from build123d import *

# Parameters (mm, degrees)
F0_W            = 25.4
F0_H            = 25.4
F1_DEPTH        = 12.7
F2_W            = 23
F2_H            = 23
F2_W_2          = 17
F2_H_2          = 17
F3_DEPTH        = 29.6
F3_COPIES_COUNT = 3
F3_COPIES_ANGLE = 180
F4_R            = 1.5


# Not quite as in the source:
# - a pattern or mirror of a feature is missing from the dataset's text; its kind, count and spacing are read off the source's solid


with BuildPart() as f1:
    # F0 (on Front) → F1 (new body, symmetric)
    with BuildSketch(Plane.XZ):
        Rectangle(F0_W, F0_H)
    extrude(amount=F1_DEPTH, both=True)

    # F2 (on face) → F3 (join)
    with BuildSketch(Plane.XZ.offset(12.7)):
        Rectangle(F2_W, F2_H)
        Rectangle(F2_W_2, F2_H_2, mode=Mode.SUBTRACT)
    f3 = extrude(amount=F3_DEPTH)

    # F3_copies: F3 ×3 about axis
    f3_copies_axis = Axis((0, 0, 0), (0, 0, 1))
    for i in range(1, F3_COPIES_COUNT):
        add(f3.rotate(f3_copies_axis, i * F3_COPIES_ANGLE / (F3_COPIES_COUNT - 1)))

    # F3_copies1: F3 across plane
    add(f3.mirror(Plane(origin=(0, 0, 0), x_dir=(0, -0.7071067812, -0.7071067812), z_dir=(0, 0.7071067812, -0.7071067812))))

    # F4
    f4_edges = [f1.edges().sort_by_distance(p)[0] for p in [
        (11.5, -27.5, 11.5),
        (11.5, -27.5, -11.5),
        (-11.5, -27.5, 11.5),
        (-11.5, -27.5, -11.5),
        (0, -42.3, 11.5),
        (11.5, -42.3, 0),
        (0, -42.3, -11.5),
        (-11.5, -42.3, 0),
        (-11.5, 27.5, -11.5),
        (-11.5, 27.5, 11.5),
        (-11.5, 42.3, 0),
        (11.5, 27.5, -11.5),
        (0, 42.3, -11.5),
        (11.5, 27.5, 11.5),
        (11.5, 42.3, 0),
        (0, 42.3, 11.5),
        (27.5, 11.5, 11.5),
        (27.5, -11.5, 11.5),
        (42.3, 0, 11.5),
        (27.5, -11.5, -11.5),
        (42.3, -11.5, 0),
        (27.5, 11.5, -11.5),
        (42.3, 0, -11.5),
        (42.3, 11.5, 0),
        (11.5, -11.5, -27.5),
        (11.5, 11.5, -27.5),
        (11.5, 0, -42.3),
        (-11.5, -11.5, -27.5),
        (0, -11.5, -42.3),
        (-11.5, 11.5, -27.5),
        (-11.5, 0, -42.3),
        (0, 11.5, -42.3),
    ]]
    fillet(f4_edges, radius=F4_R)


solid = f1.part
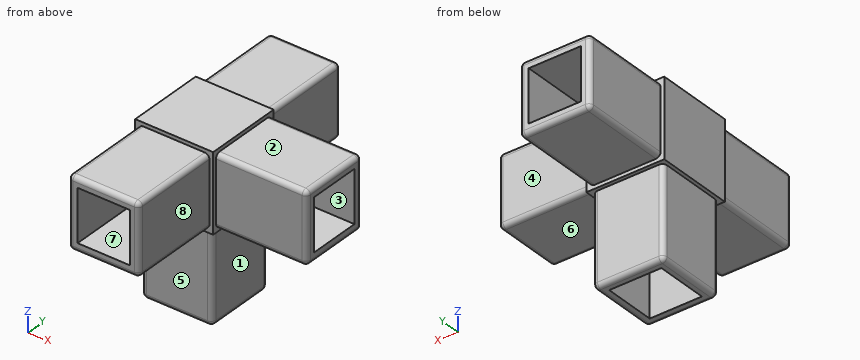
Check sheet for the modelled part. Datum: model origin and axes. Units: mm. Face numbers are marked on the shaded views. A direction names the side the tool comes from. Give positions to 0.01 mm unless a question says otherwise; leave off trailing zeros. Loops run counter-clockwise (first coordinate to the right, second up) from the corner with the lowest first, then second, coordinate; pieces in that order, holes last. Notation, with made-up numbers: M 4,80.5 L 47,80.5 A23 ccw 47,107.5 Z; hole C 60.5,-4.5 d7. An arc over 180 degrees is marked long. Return JSON: item names as keys, results as strings. Group by question number.
1. Cross-section at D-D on y = 5. Record the boundary of the cut face in (x, z), plus the area to 3 significant figures.
2. Cross-section at A-A on y = 34.5. Record the boundary of the cut face in (x, z).
3. Thickness scan on L1, parallel to Z at x = 8, y = -26.5. Record the ranges inside material, lowest first.
4. Go/stop test with flat-tipped pins: pin 1 (22 mm diameter, centred on x = 24.5, z = -0.5, fed in from -Y); pin 2 (4 mm diameter, centred on x = 0.5, z = -1, fed in from -Y); pin 3 (6 mm diameter, centred on x = 8.5, y = 19.5, fed in from -Z). Record where each tip stops, or that it passes through.
5. Tool access check on the marked faces 1, 2, 3, 4 and 5. Record the directions out of +Z, -Z, +X, -X, +Y, -Y that give a thin tool (end or side, any length) a straight path to the whole face; none if there is none.
6. Mould release check, pull along Z, two halves, no side actions. Record for the marked faces 6, 7 and 8: released by +Z, released by -Z, zero draft, split by the parting line, or undercut.
Return value:
{
 "1": {"outline": "M -12.7,-12.7 L -11.5,-12.7 L -11.5,-40.8 A1.5 ccw -10,-42.3 L -8.5,-42.3 L -8.5,-12.7 L 8.5,-12.7 L 8.5,-42.3 L 10,-42.3 A1.5 ccw 11.5,-40.8 L 11.5,-12.7 L 12.7,-12.7 L 12.7,-11.5 L 40.8,-11.5 A1.5 ccw 42.3,-10 L 42.3,-8.5 L 12.7,-8.5 L 12.7,8.5 L 42.3,8.5 L 42.3,10 A1.5 ccw 40.8,11.5 L 12.7,11.5 L 12.7,12.7 L -12.7,12.7 Z", "area": "998 mm^2"},
 "2": {"outline": "M -11.5,-10 A1.5 ccw -10,-11.5 L 10,-11.5 A1.5 ccw 11.5,-10 L 11.5,10 A1.5 ccw 10,11.5 L -10,11.5 A1.5 ccw -11.5,10 Z; hole M -8.5,-8.5 L 8.5,-8.5 L 8.5,8.5 L -8.5,8.5 Z"},
 "3": {"L1": "-11.5 to -8.5, 8.5 to 11.5"},
 "4": {"pin 1": "y = -11.5", "pin 2": "y = -12.7", "pin 3": "z = -11.5"},
 "5": {"face 1": "-Z, +X, +Y, -Y", "face 2": "+Z, +X, +Y, -Y", "face 3": "+X", "face 4": "+Z, -Z, +X, +Y", "face 5": "-Z, +X, -X, -Y"},
 "6": {"face 6": "released by -Z", "face 7": "undercut", "face 8": "zero draft"}
}
